Read the model definition and answer for the solid it produces. Units are mm, in the model's axes. A direction names the side the tool comes from. Give positions to 0.01 mm unless a question says otherwise; leave off trailing zeros. Loops run counter-clockwise (first coordinate to the right, second up) from the corner with the lowest first, then second, coordinate; pieces in that order, holes last. Notation, with made-up numbers: (74, 33.5) - (111, 33.5) arc R34 ccw to (111, 71.5) - close; hole circle Ø2 at (-1.5, -31). An arc over 180 degrees is marked (long way). Put each result on its own line as item: value. Start each with the question number.
1. Consider L1, parallel to Y at x = 1.5, z = 114.3; L2, parallel to Y at x = 7.75, z = 199 (3 decimals). Determine where each line is inside the solid, lowest interval first. Write a range as from..to.
2. A cutting plane is placed at A-A, the plane z = 17.5. Determine the outline of the cut face in (x, y) (3 decimals), plus the area to 3 significant figures.
3. For faces 1 (the flat face through (3, 5, 219.075)), 2 (the flat face through (16, 3.175, 3)), determine the directions among +Z, -Z, +X, -X, +Y, -Y from which every point of the face is accessible in a straight line to the end or side of a thin tool.
4. Given pin 1 Ø6 at (x, z) = (19.05, 206.375) entering from +Y (3 decimals); pin 2 Ø3.5 at (x, z) = (19.05, -38.1) entering from -Y; pin 3 Ø7 at (y, z) = (12.7, -214.84) entering from +X (3 decimals), each flat-ended and moving along its own axis, determine where each tip first touches the part or whether it passes through.
```python
from build123d import *

# Parameters (mm, degrees)
BOSS_EXTRUDE1_DEPTH = 219.075
FILLET1_R           = 3.175
SKETCH2_R           = 2.25
CUT_EXTRUDE1_DEPTH  = 4.175


with BuildPart() as part:
    # Sketch1 → Boss-Extrude1 (new body, symmetric)
    with BuildSketch(Plane.XY):
        Polygon((0, 25.4), (0, 0), (25.4, 0), (25.4, 3.175), (3.175, 3.175), (3.175, 25.4), align=None)
    extrude(amount=BOSS_EXTRUDE1_DEPTH, both=True)

    # Fillet1
    fillet1_edges = [part.edges().sort_by_distance(p)[0] for p in [
        (3.175, 3.175, 0),
    ]]
    fillet(fillet1_edges, radius=FILLET1_R)

    # Sketch2 → Cut-Extrude1 (cut, through all)
    with BuildSketch(Plane(origin=(3.175, 0, 0), x_dir=(0, 0, -1), z_dir=(1, 0, 0))):
        with Locations((-214.841666667, 12.7)):
            Circle(SKETCH2_R)
        with Locations((-206.375, 19.05)):
            Circle(SKETCH2_R)
        with Locations((214.841666667, 12.7)):
            Circle(SKETCH2_R)
        with Locations((206.375, 19.05)):
            Circle(SKETCH2_R)
        with Locations((-190.5, 19.05)):
            Circle(SKETCH2_R)
        with Locations((-152.4, 19.05)):
            Circle(SKETCH2_R)
        with Locations((-114.3, 19.05)):
            Circle(SKETCH2_R)
        with Locations((-76.2, 19.05)):
            Circle(SKETCH2_R)
        with Locations((-38.1, 19.05)):
            Circle(SKETCH2_R)
        with Locations((0, 19.05)):
            Circle(SKETCH2_R)
        with Locations((38.1, 19.05)):
            Circle(SKETCH2_R)
        with Locations((76.2, 19.05)):
            Circle(SKETCH2_R)
        with Locations((114.3, 19.05)):
            Circle(SKETCH2_R)
        with Locations((152.4, 19.05)):
            Circle(SKETCH2_R)
        with Locations((190.5, 19.05)):
            Circle(SKETCH2_R)
    cut_extrude1 = extrude(amount=-CUT_EXTRUDE1_DEPTH, mode=Mode.SUBTRACT)

    # Mirror1: Cut-Extrude1 across plane
    add(cut_extrude1.mirror(Plane(origin=(0, 0, 0), x_dir=(0, 0, 1), z_dir=(0.707106781, -0.707106781, 0))), mode=Mode.SUBTRACT)


solid = part.part
```
Return value:
1. L1: y = 0..16.8, 21.3..25.4
1. L2: y = 0..3.175
2. outline: (0, 0) - (25.4, 0) - (25.4, 3.175) - (6.35, 3.175) arc R3.175 cw to (3.175, 6.35) - (3.175, 25.4) - (0, 25.4) - close
2. area: 153 mm2
3. face 1: +Z, +X, -X, +Y, -Y
3. face 2: +Z, -Z, +X, +Y
4. pin 1: stops at y = 3.175
4. pin 2: passes through
4. pin 3: stops at x = 3.175
